Source: CAD feature listing. Evaluate the final solid. Frame: model axes, mm. A direction names the side the tool comes from. Coordinates: 2 decimals unless noted, no trailing zeros. Write each loop counter-clockwise with the first axis right and the second up, starting at its lowest first coordinate (ties: lowest second). Pieces come first, ordered by that corner, then holes. Notation, with made-up numbers: (11, 13) -> (42, 13) arc R31 cw to (42, 41) -> close; hole circle Ø5 at (-20, 55.25). An arc over 180 degrees is marked (long way). Write item = value, one per line.
from build123d import *

# Parameters (mm, degrees)
BOSS_EXTRUDE1_DEPTH   = 5
CUT_EXTRUDE1_REACH    = 123.758
SKETCH2_R             = 1
SKETCH2_R_2           = 1.25
CUT_EXTRUDE2_REACH    = 123.758
SKETCH3_R             = 10
SKETCH4_R             = 10
BOSS_EXTRUDE2_DEPTH   = 15
BODY_MOVE_COPY1_ANGLE = 90


with BuildPart() as part:
    # Sketch1 → Boss-Extrude1 (new body)
    with BuildSketch(Plane(origin=(0, 0, 0), x_dir=(1, 0, 0), z_dir=(0, 1, 0))):
        with BuildLine():
            Line((100, -20), (0, -20))
            ThreePointArc((0, -20), (-20, 0), (0, 20))
            Line((0, 20), (100, 20))
            ThreePointArc((100, 20), (120, 0), (100, -20))
        make_face()
    extrude(amount=BOSS_EXTRUDE1_DEPTH)

    # Sketch2 → Cut-Extrude1 (cut, up to next)
    with BuildSketch(Plane(origin=(0, 5, 0), x_dir=(1, 0, 0), z_dir=(0, 1, 0)), mode=Mode.PRIVATE) as cut_extrude1_sk1:
        with Locations(Location((0, 0, 0), (0, 0, 270))):
            Circle(SKETCH2_R)
    cut_extrude1_tool1 = extrude(cut_extrude1_sk1.sketch, amount=-CUT_EXTRUDE1_REACH, mode=Mode.PRIVATE) & part.part
    # Sketch2 → Cut-Extrude1 (cut, up to next)
    with BuildSketch(Plane(origin=(0, 5, 0), x_dir=(1, 0, 0), z_dir=(0, 1, 0)), mode=Mode.PRIVATE) as cut_extrude1_sk2:
        with Locations(Location((0, 7, 0), (0, 0, 270))):
            Circle(SKETCH2_R_2)
    cut_extrude1_tool2 = extrude(cut_extrude1_sk2.sketch, amount=-CUT_EXTRUDE1_REACH, mode=Mode.PRIVATE) & part.part
    # Sketch2 → Cut-Extrude1 (cut, up to next)
    with BuildSketch(Plane(origin=(0, 5, 0), x_dir=(1, 0, 0), z_dir=(0, 1, 0)), mode=Mode.PRIVATE) as cut_extrude1_sk3:
        with Locations(Location((7.001, 0.001, 0), (0, 0, 270))):
            Circle(SKETCH2_R_2)
    cut_extrude1_tool3 = extrude(cut_extrude1_sk3.sketch, amount=-CUT_EXTRUDE1_REACH, mode=Mode.PRIVATE) & part.part
    # Sketch2 → Cut-Extrude1 (cut, up to next)
    with BuildSketch(Plane(origin=(0, 5, 0), x_dir=(1, 0, 0), z_dir=(0, 1, 0)), mode=Mode.PRIVATE) as cut_extrude1_sk4:
        with Locations(Location((0.002, -7, 0), (0, 0, 270))):
            Circle(SKETCH2_R_2)
    cut_extrude1_tool4 = extrude(cut_extrude1_sk4.sketch, amount=-CUT_EXTRUDE1_REACH, mode=Mode.PRIVATE) & part.part
    # Sketch2 → Cut-Extrude1 (cut, up to next)
    with BuildSketch(Plane(origin=(0, 5, 0), x_dir=(1, 0, 0), z_dir=(0, 1, 0)), mode=Mode.PRIVATE) as cut_extrude1_sk5:
        with Locations(Location((-6.999, -0.001, 0), (0, 0, 270))):
            Circle(SKETCH2_R_2)
    cut_extrude1_tool5 = extrude(cut_extrude1_sk5.sketch, amount=-CUT_EXTRUDE1_REACH, mode=Mode.PRIVATE) & part.part
    add(cut_extrude1_tool1.solids().sort_by_distance((0, 5, 0))[0], mode=Mode.SUBTRACT)
    add(cut_extrude1_tool2.solids().sort_by_distance((0, 5, -7))[0], mode=Mode.SUBTRACT)
    add(cut_extrude1_tool3.solids().sort_by_distance((7.001, 5, -0.001))[0], mode=Mode.SUBTRACT)
    add(cut_extrude1_tool4.solids().sort_by_distance((0.002, 5, 7))[0], mode=Mode.SUBTRACT)
    add(cut_extrude1_tool5.solids().sort_by_distance((-6.999, 5, 0.001))[0], mode=Mode.SUBTRACT)

    # Sketch3 → Cut-Extrude2 (cut, up to next)
    with BuildSketch(Plane(origin=(0, 5, 0), x_dir=(1, 0, 0), z_dir=(0, 1, 0)), mode=Mode.PRIVATE) as cut_extrude2_sk1:
        with Locations(Location((100, 0, 0), (0, 0, 270))):
            Circle(SKETCH3_R)
    cut_extrude2_tool1 = extrude(cut_extrude2_sk1.sketch, amount=-CUT_EXTRUDE2_REACH, mode=Mode.PRIVATE) & part.part
    add(cut_extrude2_tool1.solids().sort_by_distance((100, 5, 0))[0], mode=Mode.SUBTRACT)

    # Sketch4 → Boss-Extrude2 (add)
    with BuildSketch(Plane.XZ):
        with Locations(Location((0, 0, 0), (0, 0, 90))):
            Circle(SKETCH4_R)
    extrude(amount=BOSS_EXTRUDE2_DEPTH)


with BuildPart() as part_1:
    # Body-Move/Copy1: moved
    add(part.part.rotate(Axis((0, 0, 0), (1, 0, 0)), BODY_MOVE_COPY1_ANGLE))


with BuildPart() as part_2:
    # Body-Move/Copy2: moved
    add(part_1.part.moved(Location((0, 0, -5))))


solid = part_2.part
1) Cut plane B-B, the plane x = 95.5. Output: boundary loops of the cut face in (y, z), and give its area (3 significant figures).
Answer block:
outline = (-20, -5) -> (-8.93, -5) -> (-8.93, 0) -> (-20, 0) -> close; (8.93, -5) -> (20, -5) -> (20, 0) -> (8.93, 0) -> close
area = 111 mm2
2) Cut plane A-A, the plane y = 7. Output: boundary loops of the cut face in (x, z) (3 decimals).
Answer block:
outline = (-18.735, -5) -> (-7.141, -5) -> (-7.141, -20) -> (7.141, -20) -> (7.141, -5) -> (92.859, -5) -> (92.859, 0) -> (1.25, 0) -> (1.25, -5) -> (-1.25, -5) -> (-1.25, 0) -> (-18.735, 0) -> close; (107.141, -5) -> (118.735, -5) -> (118.735, 0) -> (107.141, 0) -> close
3) Cut plane D-D, the plane x = 63. Output: boundary loops of the cut face in (y, z), and give its area (3 significant figures).
Answer block:
outline = (-20, -5) -> (20, -5) -> (20, 0) -> (-20, 0) -> close
area = 200 mm2
4) First-contact query: pin 1 Ø0.8 at (x, y) = (0, -7) entering from +Z; pin 2 Ø12 at (x, y) = (100, 0) entering from -Z; pin 3 Ø2 at (y, z) = (-12.5, -4.5) entering from +X; pin 4 Ø3 at (x, y) = (54, 9) entering from -Z. Flat tips, straight axial feed; report the tip coordinate or a pass-through.
Answer block:
pin_1 = -5
pin_2 = through
pin_3 = 116.36
pin_4 = -5
5) Material intervals for probe 1 along X at (y, z) = (0, -3.2); probe 2 along Z at (x, y) = (73.5, -0.5); probe 3 along X at (y, z) = (7, -2.1) (3 decimals), sorted ascending. Write a range as [from, to].
Answer block:
probe_1 = [-20, -8.25], [-5.75, -1], [1, 5.75], [8.25, 90], [110, 120]
probe_2 = [-5, 0]
probe_3 = [-18.735, -1.25], [1.25, 92.859], [107.141, 118.735]
6) Cut plane C-C, the plane z = -13. Output: boundary loops of the cut face in (x, y).
Answer block:
outline = circle Ø20 at (0, 0)
7) Reachability of faces 1 (the cylindrical face through (9.76, 2.17, -12.4)), 2 (the cylindrical face through (8.055, -0.671, -2.465)), 3 (the cylindrical face through (120, 0, -3)) from +Z, -Z, +X, -X, +Y, -Y: full face, straight path, thin tool, end or side. Return the list, or none.
Answer block:
face_1 = -Z
face_2 = +Z
face_3 = +Z, -Z, +X
8) Pull-direction query (Y, two-part tool) for faces 4 (the flat face through (0, 0, -20)), 5 (the flat face through (0, -7, -5)), 6 (the cylindrical face through (-20, 0, -3)); classes: +Y half, -Y half, draft (parallel to the pull), parting line (faces both ways), or undercut.
Answer block:
face_4 = draft
face_5 = undercut
face_6 = parting line
